Geometry: final body of the model. Coordinates: model frame, mm. A direction names the side the tool comes from. Give positions to 0.01 mm unless a question says otherwise; leave off trailing zeros. Write each loop counter-clockwise with the first axis right and the second up, starting at its lowest first coordinate (ties: lowest second). Pieces come first, ordered by that corner, then holes.
Autodesk Inventor part; units mm, degrees
ref_plane "Work Plane1" through (-19.05, 6.35, -76.2) normal (-1, 0, 0) x (0, 0, 1)
ref_plane "YZ Plane" through (0, 0, 0) normal (1, 0, 0) x (0, 1, 0)
ref_plane "XZ Plane" through (0, 0, 0) normal (0, 1, 0) x (-1, 0, 0)
sketch "Sketch1" plane through (0, 0, 0) normal (0, 1, 0) x (-1, 0, 0)
  line L0 (57.15, 0) -> (-19.05, 0)
  line L1 (-19.05, 0) -> (-19.05, -76.2)
  line L2 (-19.05, -76.2) -> (57.15, -76.2)
  line L3 (57.15, -76.2) -> (57.15, 0)
  point P0 (0, 0)
  dimension "d0" = 76.2
  dimension "d1" = 76.2
extrude "BOTTOM" add sketch "Sketch1" along normal blind 6.35
sketch "Sketch2" plane through (19.05, 0, -76.2) normal (0, 0, -1) x (-1, 0, 0)
  line L0 (0, 0) -> (76.2, 0)
  line L1 (76.2, 0) -> (76.2, 76.2)
  line L2 (76.2, 76.2) -> (0, 76.2)
  line L3 (0, 76.2) -> (0, 0)
  point P0 (19.05, 0)
  dimension "d4" = 76.2
  dimension "d5" = 76.2
extrude "SIDE" add sketch "Sketch2" along normal blind 6.35
sketch "Sketch3" plane through (0, 6.35, 0) normal (0, 1, 0) x (1, 0, 0)
  circle A0 centre (-19.05, 38.1) radius 9.525
  line L0 (-57.15, 76.2) -> (19.05, 76.2)
  line L1 (-57.15, 76.2) -> (-57.15, 0)
  point P0 (0, 0)
  point P1 (-44.45, 76.2)
  point P2 (6.35, 76.2)
  point P3 (-57.15, 12.7)
  dimension "d9" = 19.05
  dimension "d10" = 38.1
  dimension "d11" = 38.1
extrude "HOLE BOTT" cut sketch "Sketch3" against normal blind 6.35
sketch "Sketch4" plane through (19.05, 0, -76.2) normal (0, 0, 1) x (1, 0, 0)
  circle A0 centre (-38.1, 38.1) radius 9.525
  line L0 (-76.2, 76.2) -> (0, 76.2)
  line L1 (0, 76.2) -> (0, 6.35)
  point P0 (-19.05, 0)
  point P1 (-63.5, 76.2)
  point P2 (-12.7, 76.2)
  point P3 (0, 63.5)
  dimension "d14" = 19.05
  dimension "d15" = 38.1
  dimension "d16" = 38.1
extrude "HOLE SIDE" cut sketch "Sketch4" against normal blind 6.35
chamfer "CHM TOP" distance 12.7 angle 45 2 edges at (19.05, 76.2, -79.375) (-57.15, 76.2, -79.375)
ref_plane "Work Plane1" through (-19.05, 6.35, -76.2) normal (-1, 0, 0) x (0, 0, 1)
sketch "Sketch6" plane through (-19.05, 6.35, -76.2) normal (-1, 0, 0) x (0, 0, 1)
  line L0 (0, 0) -> (12.7, 0)
  line L1 (12.7, 0) -> (0, 12.7)
  line L2 (0, 12.7) -> (0, 0)
  point P0 (76.2, -6.35)
  dimension "d25" = 12.7
  dimension "d27" = 12.7
extrude "BRACE" add sketch "Sketch6" along normal mid plane 3.175
fillet "Fillet1" radius 10.16 2 edges at (-38.8937, 6.35, -76.2) (0.7938, 6.35, -76.2)
chamfer "CHM BOTT" distance 12.7 angle 45 2 edges at (-57.15, 3.175, 0) (19.05, 3.175, 0)
equation "\"d0\" = L"
equation "\"d1\" = w"
equation "\"d2\" = HT"
equation "\"d4\" = w"
equation "\"d5\" = L"
equation "\"d6\" = HT"
equation "\"d9\" = HL"
equation "\"d10\" = 0.5 * L"
equation "\"d11\" = 0.5 * w"
equation "\"d12\" = HT"
equation "\"d14\" = HL"
equation "\"d15\" = 0.5 * L"
equation "\"d16\" = 0.5 * w"
equation "\"d17\" = HT"
equation "\"d19\" = CHM"
equation "\"d28\" = 0.5 * HT"
equation "\"d31\" = CHM"
equation "\"d30\" = FL"
equation "\"L\" = 76.2"
equation "\"w\" = 76.2"
equation "\"HT\" = 6.35"
equation "\"CHM\" = 12.7"
equation "\"HL\" = 19.05"
equation "\"d24\" = -0.5 * w"
equation "\"FL\" = 10.16"
properties part number "PARAMETRIC L-BRAKET"
Item 1: Section A-A, the plane z = -38.1. Return the cut outline in (x, y) (3 decimals).
Found:
outline: (-57.15, 0) - (-28.575, 0) - (-28.575, 6.35) - (-57.15, 6.35) - close; (-9.525, 0) - (19.05, 0) - (19.05, 6.35) - (-9.525, 6.35) - close
Item 2: Reachability of faces 5 (the face through (-17.462, 11, -71)), 6 (the face through (-39.1, 9.4, -73.3)), 7 (the face through (-19, 0, -50)) from +Z, -Z, +X, -X, +Y, -Y: full face, straight path, thin tool, end or side. Return the list, or none.
Found:
face 5: +Z, +X, +Y
face 6: +Z, -X, +Y
face 7: +Z, -Z, +X, -X, -Y
Item 3: Section C-C, the plane x = -19.05. Return the cut outline in (y, z) (3 decimals), plus the area to 3 significant figures.
Found:
outline: (0, -82.55) - (28.575, -82.55) - (28.575, -76.2) - (19.05, -76.2) - (6.35, -63.5) - (6.35, -47.625) - (0, -47.625) - close; (0, -28.575) - (6.35, -28.575) - (6.35, 0) - (0, 0) - close; (47.625, -82.55) - (76.2, -82.55) - (76.2, -76.2) - (47.625, -76.2) - close
area: 806 mm2
Item 4: Pin query (flat end, axial travel): pin 1 Ø12 at (y, z) = (14, -53.5) entering from +X; pin 2 Ø1.5 at (x, y) = (-4, 47) entering from +Z; pin 3 Ø20 at (x, z) = (-13.5, -44.5) entering from +Y; pin 4 Ø6.5 at (y, z) = (14, -71) entering from +X. Return the tip coordinate at first contact, or that it passes through.
Found:
pin 1: passes through
pin 2: stops at z = -76.2
pin 3: stops at y = 6.35
pin 4: stops at x = -17.46
Item 5: Pull-direction query (X, two-part tool) for faces 1 (the face through (-20.29, 47.544, -79.331)), 2 (the face through (-20.29, 3.219, -47.544)), 3 (the face through (19.05, 6, -60)), 4 (the face through (-27, 30, -82.55)); classes: +X half, -X half, draft (parallel to the pull), parting line (faces both ways), or undercut.
Found:
face 1: undercut
face 2: undercut
face 3: +X half
face 4: draft
Item 6: Section B-B, the plane y = 38.1. Return the cut outline in (x, z) (3 decimals), plus the area to 3 significant figures.
Found:
outline: (-57.15, -82.55) - (-28.575, -82.55) - (-28.575, -76.2) - (-57.15, -76.2) - close; (-9.525, -82.55) - (19.05, -82.55) - (19.05, -76.2) - (-9.525, -76.2) - close
area: 363 mm2
Item 7: Section D-D, the plane z = -73.5. Return the cut outline in (x, y).
Found:
outline: (-57.15, 0) - (19.05, 0) - (19.05, 9.61) - (-17.46, 9.61) - (-17.46, 16.35) - (-20.64, 16.35) - (-20.64, 9.61) - (-57.15, 9.61) - close
Item 8: Line query: L1, parallel to X at y = 1, z = -38; L2, parallel to Y at x = -19, z = -79; L3, parallel to Z at x = -19.05, y = 1.5 (3 decimals). Output: solid intervals per line, ascending.
Found:
L1: x = -57.15 to -28.57, -9.53 to 19.05
L2: y = 0 to 28.58, 47.62 to 76.2
L3: z = -82.55 to -47.625, -28.575 to 0
